```python
from build123d import *

# Parameters (mm, degrees)
SKETCH1_W           = 40
SKETCH1_H           = 40
BOSS_EXTRUDE1_DEPTH = 3.4
SKETCH2_R           = 0.5
BOSS_EXTRUDE2_DEPTH = 12.7
SKETCH3_R           = 0.4953
BOSS_EXTRUDE3_DEPTH = 12.7


with BuildPart() as part:
    # Sketch1 → Boss-Extrude1 (new body)
    with BuildSketch(Plane(origin=(0, 0, 0), x_dir=(1, 0, 0), z_dir=(0, 1, 0))):
        with Locations((-30.671871438, 7.059468761)):
            Rectangle(SKETCH1_W, SKETCH1_H)
    extrude(amount=BOSS_EXTRUDE1_DEPTH)

    # Sketch2 → Boss-Extrude2 (add)
    with BuildSketch(Plane(origin=(0, 0, -27.059468761), x_dir=(-1, 0, 0), z_dir=(0, 0, -1))):
        with Locations((48.671871438, 1.7)):
            Circle(SKETCH2_R)
    extrude(amount=BOSS_EXTRUDE2_DEPTH)

    # Sketch3 → Boss-Extrude3 (add)
    with BuildSketch(Plane(origin=(0, 0, -27.059468761), x_dir=(-1, 0, 0), z_dir=(0, 0, -1))):
        with Locations((12.678471438, 1.772009117)):
            Circle(SKETCH3_R)
    extrude(amount=BOSS_EXTRUDE3_DEPTH)


solid = part.part
```
The model under review builds one solid part; all positions refer to its coordinate system, in mm. A direction names the side the tool comes from. Round coordinates to 2 decimals unless told otherwise and drop trailing zeros. Loops run counter-clockwise (first coordinate to the right, second up) from the corner with the lowest first, then second, coordinate; pieces in that order, holes last. Notation, with made-up numbers: (-32.75, 28) - (18.25, 28) arc R25 ccw to (18.25, 56) - close; hole circle Ø7 at (53.5, 47.25). An arc over 180 degrees is marked (long way). Write each question's results on one line, items separated by ' | '. Start each with the question number.
Q1. Take a section at B-B on x = -44.5. Give the boundary of the cut face in (y, z), plus the area to 3 significant figures.
Q2. Draft analysis for pull direction X (two halves, no side actions). For faces 1 (the flat face through (-50.672, 2, -7)), 2 (the flat face through (-31, 0, -7)), 3 (the flat face through (-10.672, 2, -7)), 4 (the flat face through (-31, 2, -27.059)), state which applies: pulls with the +X half, pulls with the -X half, needs draft (parallel to the pull), parting line crosses it, or undercut.
Q3. Insertion check: P1, Ø1, axis at x = -36, y = 1.5, coming from the -Z side. The pin has a flat end and moves straight along its axis. Give the tip position at first contact, or say it passes through.
Q4. Tool access review of faces 5 (the flat face through (-31, 2, 12.941)), 6 (the cylindrical face through (-48.172, 1.722, -33.321)): name each direction out of +Z, -Z, +X, -X, +Y, -Y from which nothing blocks a thin tool from reaching the whole face with its end or side.
Q5. Wall thickness on line 1 along Z through (x, y) = (-23, 0.7); line 2 along X through (y, z) = (1.9, -32): over which ranges is each line inside the solid? List them lowest first. Write a range as [from, to].
Q6. Take a section at A-A on z = -29. Give the boundary of the cut face in (x, y), plus the area to 3 significant figures.
Data:
1) outline: (0, -27.06) - (3.4, -27.06) - (3.4, 12.94) - (0, 12.94) - close | area: 136 mm²
2) face 1: pulls with the -X half | face 2: needs draft | face 3: pulls with the +X half | face 4: undercut
3) P1: stops at z = -27.06
4) face 5: +Z, +X, -X, +Y, -Y | face 6: -Z
5) line 1: z = [-27.06, 12.94] | line 2: x = [-49.13, -48.21], [-13.16, -12.2]
6) outline: circle Ø1 at (-48.67, 1.7); circle Ø0.99 at (-12.68, 1.77) | area: 1.56 mm²
